Design review of the part built by this model. Coordinates are the model's own, in mm. Give positions to 0.01 mm unless a question says otherwise; leave off trailing zeros. Order: outer loops, then holes, each group sorted by start corner. A loop starts at its lowest first (then second) coordinate and runs counter-clockwise, first axis right, second up.
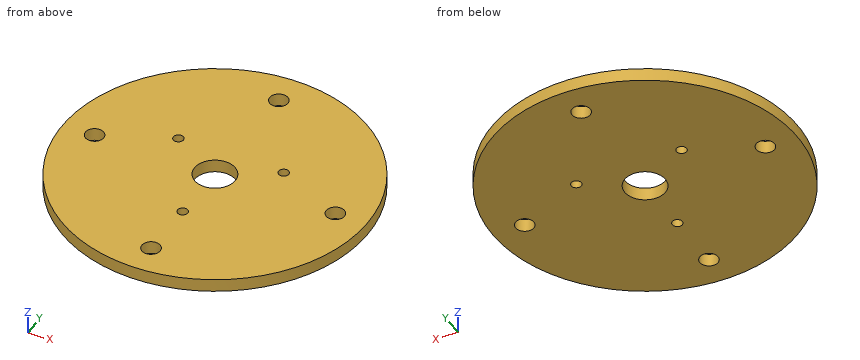
```python
from build123d import *

# Parameters (mm, degrees)
SKETCH1_R           = 37.5
SKETCH1_R_2         = 2.25
SKETCH1_R_3         = 5
SKETCH1_R_4         = 1.25
BOSS_EXTRUDE1_DEPTH = 3.2


with BuildPart() as part:
    # Sketch1 → Boss-Extrude1 (new body)
    with BuildSketch(Plane.XY):
        Circle(SKETCH1_R)
        with Locations((0, 29.7)):
            Circle(SKETCH1_R_2, mode=Mode.SUBTRACT)
        Circle(SKETCH1_R_3, mode=Mode.SUBTRACT)
        with Locations((29.7, 0)):
            Circle(SKETCH1_R_2, mode=Mode.SUBTRACT)
        with Locations((0, -29.7)):
            Circle(SKETCH1_R_2, mode=Mode.SUBTRACT)
        with Locations((-29.7, 0)):
            Circle(SKETCH1_R_2, mode=Mode.SUBTRACT)
        with Locations((-12.990381057, 7.5)):
            Circle(SKETCH1_R_4, mode=Mode.SUBTRACT)
        with Locations((12.990381057, 7.5)):
            Circle(SKETCH1_R_4, mode=Mode.SUBTRACT)
        with Locations((0, -15)):
            Circle(SKETCH1_R_4, mode=Mode.SUBTRACT)
    extrude(amount=BOSS_EXTRUDE1_DEPTH)


solid = part.part
```
1. Take a section at A-A (z = 2.4). State how many separate pieces and enclosed holes the cut face has, then the cut area to 3 significant figures.
Recorded:
separate pieces: 1
enclosed holes: 8
area: 4,260 mm2
2. Take a section at D-D (y = 7.5). State the section outline as (x, z) points, then the cut area to 3 significant figures.
Recorded:
outline: (-36.74, 0) - (-14.24, 0) - (-14.24, 3.2) - (-36.74, 3.2) - close; (-11.74, 0) - (11.74, 0) - (11.74, 3.2) - (-11.74, 3.2) - close; (14.24, 0) - (36.74, 0) - (36.74, 3.2) - (14.24, 3.2) - close
area: 219 mm2
3. For pin 1 (1 mm diameter, centred on y = 2.5, z = 1, fed in from +X); pin 2 (1 mm diameter, centred on x = -13.5, z = 2.5, fed in from +Y), all flat-tipped, find the tip position at first contact; note any pin that passes through.
Recorded:
pin 1: stops at x = 37.45
pin 2: stops at y = 35.17
4. Take a section at B-B (y = -29.7). State the section outline as (x, z) points, then the cut area to 3 significant figures.
Recorded:
outline: (-22.89, 0) - (-2.25, 0) - (-2.25, 3.2) - (-22.89, 3.2) - close; (2.25, 0) - (22.89, 0) - (22.89, 3.2) - (2.25, 3.2) - close
area: 132 mm2
5. For line 1 along Y through (x, z) = (0, 1.6); line 2 along Y through (x, z) = (0.5, 2.65); line 3 along Y through (x, z) = (2, 1.75), list the stretches that pass through material, from the lowest coordinate up.
Recorded:
line 1: y = -37.5 to -31.95, -27.45 to -16.25, -13.75 to -5, 5 to 27.45, 31.95 to 37.5
line 2: y = -37.5 to -31.89, -27.51 to -16.15, -13.85 to -4.97, 4.97 to 27.51, 31.89 to 37.5
line 3: y = -37.45 to -30.73, -28.67 to -4.58, 4.58 to 28.67, 30.73 to 37.45
